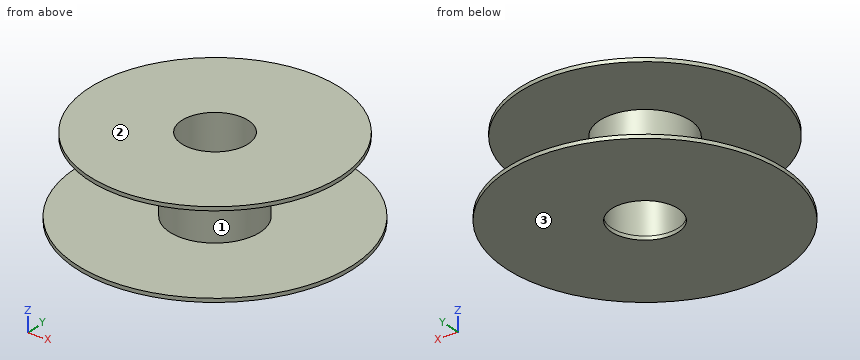
from build123d import *

# Parameters (mm, degrees)
SKETCH1_R           = 36
SKETCH1_R_2         = 26.5
EXTRUDE1_DEPTH      = 29.1
EXTRUDE1_DEPTH_BACK = 29.1
SKETCH2_R           = 100
SKETCH2_R_2         = 26.5
EXTRUDE4_DEPTH      = 3
SKETCH4_R           = 110
SKETCH4_R_2         = 26.5
EXTRUDE5_DEPTH      = 3


with BuildPart() as part:
    # Sketch1 → Extrude1 (new body, two sides)
    with BuildSketch(Plane.XY) as extrude1_sk:
        Circle(SKETCH1_R)
        Circle(SKETCH1_R_2, mode=Mode.SUBTRACT)
    extrude(amount=EXTRUDE1_DEPTH)
    extrude(extrude1_sk.sketch, amount=-EXTRUDE1_DEPTH_BACK)

    # Sketch2 → Extrude4 (add)
    with BuildSketch(Plane.XY.offset(29.1)):
        Circle(SKETCH2_R)
        Circle(SKETCH2_R_2, mode=Mode.SUBTRACT)
    extrude(amount=EXTRUDE4_DEPTH)

    # Sketch4 → Extrude5 (add)
    with BuildSketch(Plane(origin=(0, 0, -29.1), x_dir=(-1, 0, 0), z_dir=(0, 0, -1))):
        Circle(SKETCH4_R)
        Circle(SKETCH4_R_2, mode=Mode.SUBTRACT)
    extrude(amount=EXTRUDE5_DEPTH)


solid = part.part
Read the model definition and answer for the solid it produces. Units are mm, in the model's axes. Face numbers are marked on the shaded views. Round coordinates to 2 decimals unless told otherwise and drop trailing zeros. Write each loop counter-clockwise with the first axis right and the second up, starting at its lowest first coordinate (ties: lowest second). Pieces come first, ordered by that corner, then holes. Notation, with made-up numbers: (15.25, 72) - (29.25, 72) arc R27 ccw to (29.25, 109) - close; hole circle Ø4 at (81.25, 27). An arc over 180 degrees is marked (long way). One line per question, with ' | ' between items. Start each with the question number.
1. For a pull along Z with two mould halves and no side action, classify the marked faces 1, 2 and 3 as +Z half, -Z half, draft (parallel to the pull), parting line (faces both ways), or undercut.
2. Section A-A (y = 0) is taken. Determine the outline of the cut face in (x, z), and give its area (3 significant figures).
3. Section D-D (z = -7.5) is taken. Determine the outline of the cut face in (x, y), and give its area (3 significant figures).
4. This flat-tipped pin is pushed along its axis until it touches: pin 1 (4 mm diameter, centred on x = 25, z = -1, fed in from +Y). Where does it stop, or does it pass through?
5. Find the intervals of material crossed by probe 1 along Y at (x, z) = (0, 0); probe 2 along Z at (x, y) = (-8.5, -50.5); probe 3 along Y at (x, z) = (-20, -16.5), in increasing order. Write a range as [from, to].
6. Section C-C (y = -31) is taken. Determine the outline of the cut face in (x, z), and give its area (3 significant figures).
Filled in:
1) face 1: undercut | face 2: +Z half | face 3: -Z half
2) outline: (-110, -32.1) - (-26.5, -32.1) - (-26.5, 32.1) - (-100, 32.1) - (-100, 29.1) - (-36, 29.1) - (-36, -29.1) - (-110, -29.1) - close; (26.5, -32.1) - (110, -32.1) - (110, -29.1) - (36, -29.1) - (36, 29.1) - (100, 29.1) - (100, 32.1) - (26.5, 32.1) - close | area: 2,050 mm²
3) outline: circle Ø72 at (0, 0); hole circle Ø53 at (0, 0) | area: 1,870 mm²
4) pin 1: y = 27.69
5) probe 1: [-36, -26.5], [26.5, 36] | probe 2: [-32.1, -29.1], [29.1, 32.1] | probe 3: [-29.93, -17.39], [17.39, 29.93]
6) outline: (-105.54, -32.1) - (105.54, -32.1) - (105.54, -29.1) - (18.3, -29.1) - (18.3, 29.1) - (95.07, 29.1) - (95.07, 32.1) - (-95.07, 32.1) - (-95.07, 29.1) - (-18.3, 29.1) - (-18.3, -29.1) - (-105.54, -29.1) - close | area: 3,330 mm²
